```python
from build123d import *

# Parameters (mm, degrees)
SKETCH1_W           = 49.53
SKETCH1_H           = 28.575
SKETCH1_R           = 2.2225
BOSS_EXTRUDE1_DEPTH = 3.175
SKETCH2_W           = 49.53
SKETCH2_H           = 3.175
BOSS_EXTRUDE2_DEPTH = 25.4
SKETCH4_R           = 2.54
CUT_EXTRUDE1_DEPTH  = 3.175
SKETCH5_W           = 15.24
SKETCH5_H           = 28.575
CUT_EXTRUDE2_DEPTH  = 3.175
FILLET2_R           = 1.27


with BuildPart() as part:
    # Sketch1 → Boss-Extrude1 (new body)
    with BuildSketch(Plane(origin=(0, 0, 0), x_dir=(1, 0, 0), z_dir=(0, 1, 0))):
        with Locations((24.765, 14.2875)):
            Rectangle(SKETCH1_W, SKETCH1_H)
        with Locations(Location((23.495, 15.875, 0), (0, 0, 270))):
            Circle(SKETCH1_R, mode=Mode.SUBTRACT)
        with Locations(Location((43.815, 15.875, 0), (0, 0, 270))):
            Circle(SKETCH1_R, mode=Mode.SUBTRACT)
    extrude(amount=BOSS_EXTRUDE1_DEPTH)

    # Sketch2 → Boss-Extrude2 (add)
    with BuildSketch(Plane(origin=(0, 3.175, 0), x_dir=(1, 0, 0), z_dir=(0, 1, 0))):
        with Locations((24.765, 1.5875)):
            Rectangle(SKETCH2_W, SKETCH2_H)
    extrude(amount=BOSS_EXTRUDE2_DEPTH)

    # Sketch4 → Cut-Extrude1 (cut)
    with BuildSketch(Plane(origin=(0, 0, -3.175), x_dir=(-1, 0, 0), z_dir=(0, 0, -1))):
        with Locations((-12.065, 15.875)):
            Circle(SKETCH4_R)
        with Locations((-37.465, 15.875)):
            Circle(SKETCH4_R)
    extrude(amount=-CUT_EXTRUDE1_DEPTH, mode=Mode.SUBTRACT)

    # Sketch5 → Cut-Extrude2 (cut)
    with BuildSketch(Plane.XZ):
        with Locations((7.62, -14.2875)):
            Rectangle(SKETCH5_W, SKETCH5_H)
    extrude(amount=-CUT_EXTRUDE2_DEPTH, mode=Mode.SUBTRACT)

    # Fillet2
    fillet2_edges = [part.edges().sort_by_distance(p)[0] for p in [
        (32.385, 3.175, -3.175),
    ]]
    fillet(fillet2_edges, radius=FILLET2_R)


solid = part.part
```
The listing builds one solid part. Answer for the finished solid, in the listing's coordinates (mm). A direction names the side the tool comes from. Round coordinates to 2 decimals unless told otherwise and drop trailing zeros. Write each loop counter-clockwise with the first axis right and the second up, starting at its lowest first coordinate (ties: lowest second). Pieces come first, ordered by that corner, then holes. Notation, with made-up numbers: (10.5, 40.25) -> (65.5, 40.25) arc R17 ccw to (65.5, 72.25) -> close; hole circle Ø2 at (32, -6). An arc over 180 degrees is marked (long way). Answer as a JSON object with one key per item and string values. Group by question number.
Q1. Section D-D (y = 8.25) is taken. Write down the section's boundary in (x, z) (3 decimals), plus the area to 3 significant figures.
Q2. Section A-A (x = 22) is taken. Write down the section's boundary in (y, z) (3 decimals), plus the area to 3 significant figures.
Q3. Section C-C (z = -6.25) is taken. Write down the section's boundary in (x, y) (3 decimals).
Q4. Straight lines are drawn through the part: line 1 along X through (y, z) = (3, -15.75); line 2 along Y through (x, z) = (37, -7.5) (3 decimals); line 3 along Z through (x, y) = (20, 4.75) (3 decimals). For each, find the intervals that lie inside material, in ascending order.
Q5. Section B-B (x = 17) is taken. Write down the section's boundary in (y, z) (3 decimals), plus the area to 3 significant figures.
Q6. Which of the six approach directions +Z, -Z, +X, -X, +Y, -Y give full straight-line access (tool end or side, diameter ignored) to faces 4 (the face through (32, 3.175, -17)), 5 (the face through (41.843, 1.565, -14.849)), 6 (the face through (8, 3.175, -2))?
Q7. Determine the mould class of faces 1 (the face through (24.163, 1.565, -13.755)), 2 (the face through (32, 2, -28.575)), 3 (the face through (49.53, 8, -3)) for opening direction Z: pulls with the +Z half, pulls with the -Z half, needs draft (parallel to the pull), parting line crosses it, or undercut.
Q8. Each of these flat-tipped pins is pushed along its axis until it touches: pin 1 Ø8 at (x, z) = (15, -23.5) entering from +Y (3 decimals); pin 2 Ø3.5 at (x, z) = (6.5, -2) entering from -Y (3 decimals); pin 3 Ø12.5 at (x, y) = (19, 11.5) entering from -Z (3 decimals); pin 4 Ø4 at (x, y) = (12.065, 15.875) entering from -Z. Where does it stop, or does it pass through?
Check values:
{
 "1": {"outline": "(0, -3.175) -> (49.53, -3.175) -> (49.53, 0) -> (0, 0) -> close", "area": "157 mm^2"},
 "2": {"outline": "(0, -28.575) -> (3.175, -28.575) -> (3.175, -17.52) -> (0, -17.52) -> close; (0, -14.23) -> (3.175, -14.23) -> (3.175, -4.445) arc R1.27 cw to (4.445, -3.175) -> (28.575, -3.175) -> (28.575, 0) -> (0, 0) -> close", "area": "161 mm^2"},
 "3": {"outline": "(15.24, 0) -> (49.53, 0) -> (49.53, 3.175) -> (15.24, 3.175) -> close"},
 "4": {"line 1": "15.24 to 21.28, 25.71 to 41.6, 46.03 to 49.53", "line 2": "0 to 3.175", "line 3": "-3.175 to 0"},
 "5": {"outline": "(0, -28.575) -> (3.175, -28.575) -> (3.175, -4.445) arc R1.27 cw to (4.445, -3.175) -> (28.575, -3.175) -> (28.575, 0) -> (0, 0) -> close", "area": "172 mm^2"},
 "6": {"face 4": "-Z, +X, -X, +Y", "face 5": "+Y, -Y", "face 6": "+Z, -Z, -X, -Y"},
 "7": {"face 1": "undercut", "face 2": "pulls with the -Z half", "face 3": "needs draft"},
 "8": {"pin 1": "y = 3.175", "pin 2": "y = 3.175", "pin 3": "z = -3.175", "pin 4": "through"}
}
